from build123d import *

# Parameters (mm, degrees)
ESQUISSE1_W                = 210.950231097
ESQUISSE1_H                = 93.600386247
BOSS_EXTRU_1_DEPTH         = 5
ENL_V_MAT_EXTRU_1_DEPTH    = 5
ESQUISSE4_W                = 5
ESQUISSE4_H                = 10
ENL_V_MAT_EXTRU_2_DEPTH    = 5
R_P_TITION_LIN_AIRE1_COUNT = 5
R_P_TITION_LIN_AIRE1_PITCH = 15
ESQUISSE5_W                = 17.5
ESQUISSE5_H                = 5
ENL_V_MAT_EXTRU_3_DEPTH    = 5
R_P_TITION_LIN_AIRE2_COUNT = 7
R_P_TITION_LIN_AIRE2_PITCH = 27.5
ENL_V_MAT_EXTRU_4_DEPTH    = 5
ESQUISSE8_R                = 10.303452194
ESQUISSE8_R_2              = 16.92457318
ESQUISSE8_R_3              = 12.058004818
ESQUISSE8_R_4              = 20.840400714
ESQUISSE8_R_5              = 14.375020811
ENL_V_MAT_EXTRU_5_DEPTH    = 5
SYM_TRIE1_COPY_1_SKETCH_W  = 5
SYM_TRIE1_COPY_1_SKETCH_H  = 10
SYM_TRIE1_COPY_1_DEPTH     = 5
SYM_TRIE1_COPY_2_SKETCH_W  = 5
SYM_TRIE1_COPY_2_SKETCH_H  = 10
SYM_TRIE1_COPY_2_DEPTH     = 5
SYM_TRIE1_COPY_3_SKETCH_W  = 5
SYM_TRIE1_COPY_3_SKETCH_H  = 10
SYM_TRIE1_COPY_3_DEPTH     = 5
SYM_TRIE1_COPY_4_SKETCH_W  = 5
SYM_TRIE1_COPY_4_SKETCH_H  = 10
SYM_TRIE1_COPY_4_DEPTH     = 5
ESQUISSE9_W                = 5
ESQUISSE9_H                = 3.1
ENL_V_MAT_EXTRU_6_DEPTH    = 15
ENL_V_MAT_EXTRU_7_DEPTH    = 15


with BuildPart() as part:
    # Esquisse1 → Boss.-Extru.1 (new body)
    with BuildSketch(Plane(origin=(163.933470491, 0, 0), x_dir=(0, 0, -1), z_dir=(1, 0, 0))):
        with Locations((-399.975115549, 32.112736727)):
            Rectangle(ESQUISSE1_W, ESQUISSE1_H)
    extrude(amount=-BOSS_EXTRU_1_DEPTH)

    # Esquisse3 → Enl_v. mat.-Extru.1 (cut)
    with BuildSketch(Plane(origin=(163.933470491, 0, 0), x_dir=(0, 0, -1), z_dir=(1, 0, 0))):
        Polygon((-505.450231097, -14.687456397), (-294.5, -1.08707015), (-294.5, -1.14043518), (-294.5, -14.687456397), align=None)
    extrude(amount=-ENL_V_MAT_EXTRU_1_DEPTH, mode=Mode.SUBTRACT)

    # Esquisse4 → Enl_v. mat.-Extru.2 (cut)
    with BuildSketch(Plane(origin=(163.933470491, 0, 0), x_dir=(0, 0, -1), z_dir=(1, 0, 0))):
        with Locations((-297, 8.91292985)):
            Rectangle(ESQUISSE4_W, ESQUISSE4_H)
    enl_v_mat_extru_2 = extrude(amount=-ENL_V_MAT_EXTRU_2_DEPTH, mode=Mode.SUBTRACT)

    # R_p_tition lin_aire1: Enl_v. mat.-Extru.2 ×5
    with Locations(*[(0, i * R_P_TITION_LIN_AIRE1_PITCH, 0) for i in range(1, R_P_TITION_LIN_AIRE1_COUNT)]):
        add(enl_v_mat_extru_2, mode=Mode.SUBTRACT)

    # Esquisse5 → Enl_v. mat.-Extru.3 (cut)
    with BuildSketch(Plane(origin=(163.933470491, 0, 0), x_dir=(0, 0, -1), z_dir=(1, 0, 0))):
        with Locations((-318.25, 76.41292985)):
            Rectangle(ESQUISSE5_W, ESQUISSE5_H)
    enl_v_mat_extru_3 = extrude(amount=-ENL_V_MAT_EXTRU_3_DEPTH, mode=Mode.SUBTRACT)

    # R_p_tition lin_aire2: Enl_v. mat.-Extru.3 ×7
    with Locations(*[(0, 0, i * R_P_TITION_LIN_AIRE2_PITCH) for i in range(1, R_P_TITION_LIN_AIRE2_COUNT)]):
        add(enl_v_mat_extru_3, mode=Mode.SUBTRACT)

    # Esquisse6 → Enl_v. mat.-Extru.4 (cut)
    with BuildSketch(Plane(origin=(163.933470491, 0, 0), x_dir=(0, 0, -1), z_dir=(1, 0, 0))):
        Polygon((-492, 73.91292985), (-505.450231097, 70.214096677), (-505.450231097, 78.91292985), (-492, 78.91292985), align=None)
    extrude(amount=-ENL_V_MAT_EXTRU_4_DEPTH, mode=Mode.SUBTRACT)

    # Esquisse8 → Enl_v. mat.-Extru.5 (cut)
    with BuildSketch(Plane(origin=(163.933470491, 0, 0), x_dir=(0, 0, -1), z_dir=(1, 0, 0))):
        with Locations((-357.495437595, 26.166642192)):
            Circle(ESQUISSE8_R)
        with Locations((-329.552133235, 48.980591934)):
            Circle(ESQUISSE8_R_2)
        with Locations((-390.585162306, 54.491117128)):
            Circle(ESQUISSE8_R_3)
        with Locations((-424.160939117, 18.322009653)):
            Circle(ESQUISSE8_R_4)
        with Locations((-466.318690215, 46.435552099)):
            Circle(ESQUISSE8_R_5)
    extrude(amount=-ENL_V_MAT_EXTRU_5_DEPTH, mode=Mode.SUBTRACT)

    # Sym_trie1: Enl_v. mat.-Extru.2 across plane
    add(enl_v_mat_extru_2.mirror(Plane(origin=(0, 0, 399.975115549), x_dir=(1, 0, 0), z_dir=(0, 0, -1))), mode=Mode.SUBTRACT)

    # Sym_trie1 copy 1 sketch → Sym_trie1 copy 1 (cut)
    with BuildSketch(Plane(origin=(163.933470491, 15, 799.950231097), x_dir=(0, 0, 1), z_dir=(1, 0, 0))):
        with Locations((-297, -8.91292985)):
            Rectangle(SYM_TRIE1_COPY_1_SKETCH_W, SYM_TRIE1_COPY_1_SKETCH_H)
    extrude(amount=-SYM_TRIE1_COPY_1_DEPTH, mode=Mode.SUBTRACT)

    # Sym_trie1 copy 2 sketch → Sym_trie1 copy 2 (cut)
    with BuildSketch(Plane(origin=(163.933470491, 30, 799.950231097), x_dir=(0, 0, 1), z_dir=(1, 0, 0))):
        with Locations((-297, -8.91292985)):
            Rectangle(SYM_TRIE1_COPY_2_SKETCH_W, SYM_TRIE1_COPY_2_SKETCH_H)
    extrude(amount=-SYM_TRIE1_COPY_2_DEPTH, mode=Mode.SUBTRACT)

    # Sym_trie1 copy 3 sketch → Sym_trie1 copy 3 (cut)
    with BuildSketch(Plane(origin=(163.933470491, 45, 799.950231097), x_dir=(0, 0, 1), z_dir=(1, 0, 0))):
        with Locations((-297, -8.91292985)):
            Rectangle(SYM_TRIE1_COPY_3_SKETCH_W, SYM_TRIE1_COPY_3_SKETCH_H)
    extrude(amount=-SYM_TRIE1_COPY_3_DEPTH, mode=Mode.SUBTRACT)

    # Sym_trie1 copy 4 sketch → Sym_trie1 copy 4 (cut)
    with BuildSketch(Plane(origin=(163.933470491, 60, 799.950231097), x_dir=(0, 0, 1), z_dir=(1, 0, 0))):
        with Locations((-297, -8.91292985)):
            Rectangle(SYM_TRIE1_COPY_4_SKETCH_W, SYM_TRIE1_COPY_4_SKETCH_H)
    extrude(amount=-SYM_TRIE1_COPY_4_DEPTH, mode=Mode.SUBTRACT)

    # Esquisse9 → Enl_v. mat.-Extru.6 (cut)
    with BuildSketch(Plane(origin=(0, 17.825842347, 1.149267957), x_dir=(1, 0, 0), z_dir=(0, -0.9979281364682809, -0.06433843676173626))):
        with Locations((161.433470491, 483.588677553)):
            Rectangle(ESQUISSE9_W, ESQUISSE9_H)
    extrude(amount=-ENL_V_MAT_EXTRU_6_DEPTH, mode=Mode.SUBTRACT)

    # Esquisse10 → Enl_v. mat.-Extru.7 (cut)
    with BuildSketch(Plane(origin=(163.933470491, 0, 0), x_dir=(0, 0, -1), z_dir=(1, 0, 0))):
        Polygon((-485.612619151, -8.271594794), (-489.604331697, -8.528948541), (-489.926023881, -3.539307858), (-485.934311335, -3.281954111), align=None)
    enl_v_mat_extru_7 = extrude(amount=-ENL_V_MAT_EXTRU_7_DEPTH, mode=Mode.SUBTRACT)

    # Sym_trie2: Enl_v. mat.-Extru.7 across plane
    add(enl_v_mat_extru_7.mirror(Plane(origin=(0, -31.113339549, 482.586747808), x_dir=(1, 0, 0), z_dir=(0, 0.06433843676173628, -0.997928136468281))), mode=Mode.SUBTRACT)


solid = part.part
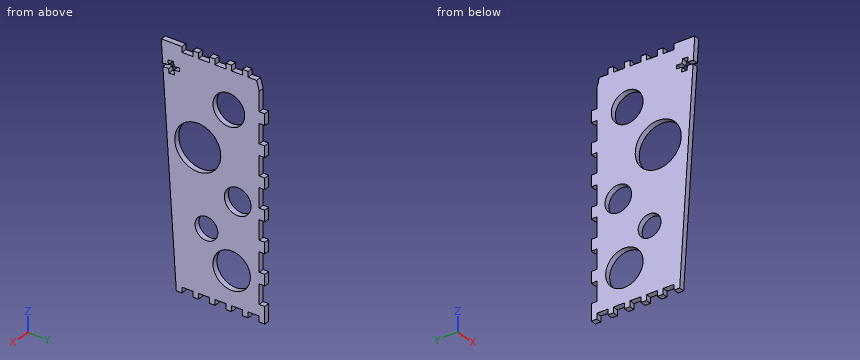
Model file for the job. Use its own axes, mm. Round coordinates to 2 decimals unless told otherwise and drop trailing zeros. Order: outer loops, then holes, each group sorted by start corner. A loop starts at its lowest first (then second) coordinate and runs counter-clockwise, first axis right, second up.
(1) Band-saw the part on B-B (z = 316.5). List the corners of the cut face in (x, y), then the cut area to 3 significant figures.
(2) Band-saw the part on D-D (z = 389.5). List the corners of the cut face in (x, y).
(3) Pin check, flat tips, straight feed: pin 1 (1.5 mm diameter, centred on x = 160, z = 297, fed in from -Y); pin 2 (2.5 mm diameter, centred on x = 160.5, z = 502, fed in from -Y); pin 3 (3 mm diameter, centred on x = 162, z = 396.5, fed in from +Y). Stop position of each tip, or through.
(4) Drill centre lines: line 1 (Z direction, x = 160.05, y = 19.5); line 2 (Z direction, x = 162.2, y = 61.5); line 3 (Y direction, x = 162.75, z = 428). Where is each one in solid material? Low to high.
(5) Band-saw the part on C-C (x = 161.6). Give the number of separate pieces and of enclosed holes in the cut face, then the cut area to 3 significant figures.
(6) Band-saw the part on A-A (y = 21.5). List the corners of the cut face in (x, z).
Verdict:
1. outline: (158.93, -2.51) - (163.93, -2.51) - (163.93, 38.21) - (158.93, 38.21) - close; (158.93, 59.75) - (163.93, 59.75) - (163.93, 73.91) - (158.93, 73.91) - close
1. area: 274 mm2
2. outline: (158.93, -7.21) - (163.93, -7.21) - (163.93, 42.48) - (158.93, 42.48) - close; (158.93, 66.5) - (163.93, 66.5) - (163.93, 78.91) - (158.93, 78.91) - close
3. pin 1: stops at y = -1.3
3. pin 2: stops at y = -14.55
3. pin 3: stops at y = 73.91
4. line 1: z = 299.5 to 349.64, 365.35 to 403.35, 444.97 to 500.45
4. line 2: z = 294.5 to 318.16, 340.94 to 380.77, 400.4 to 505.45
4. line 3: y = -9.69 to -2.16, 38.81 to 73.91
5. separate pieces: 1
5. enclosed holes: 5
5. area: 13,300 mm2
6. outline: (158.93, 299.5) - (163.93, 299.5) - (163.93, 348.31) - (158.93, 348.31) - close; (158.93, 366.68) - (163.93, 366.68) - (163.93, 403.56) - (158.93, 403.56) - close; (158.93, 444.76) - (163.93, 444.76) - (163.93, 500.45) - (158.93, 500.45) - close
